For this review, take the finished solid that the model builds, in its own axes (mm). A direction names the side the tool comes from. Give positions to 0.01 mm unless a question says otherwise; leave off trailing zeros. Loops run counter-clockwise (first coordinate to the right, second up) from the corner with the lowest first, then second, coordinate; pieces in that order, holes last.
```python
from build123d import *

# Parameters (mm, degrees)
BASE_FLANGE1_START = -58.5
BASE_FLANGE1_DEPTH = 58.5
SKETCH7_R          = 3.2
CUT_EXTRUDE1_DEPTH = 75.505788366
SKETCH8_R          = 4.45
CUT_EXTRUDE2_DEPTH = 75.505788366


# Read off the part's stored shape, not the designer's step: Base-Flange1
with BuildPart() as part:
    # Base-Flange1 outline → Base-Flange1 (new body)
    with BuildSketch(Plane.XY.offset(BASE_FLANGE1_START)):
        with BuildLine():
            ThreePointArc((9.9634, 0), (11.7924024, 0.7575976), (12.55, 2.5866))
            Line((12.55, 2.5866), (12.55, 44.4))
            Line((12.55, 44.4), (10.7, 44.4))
            Line((10.7, 44.4), (10.7, 2.5866))
            ThreePointArc((10.7, 2.5866), (10.484254855, 2.065745145), (9.9634, 1.85))
            Line((9.9634, 1.85), (0, 1.85))
            Line((0, 1.85), (0, 0))
            Line((0, 0), (9.9634, 0))
        make_face()
    extrude(amount=BASE_FLANGE1_DEPTH)

    # Sketch7 → Cut-Extrude1 (cut, through all)
    with BuildSketch(Plane(origin=(0, 0, 0), x_dir=(0, 0, -1), z_dir=(1, 0, 0))):
        with BuildLine():
            Line((11.941667032, 43.361555933), (58.5, 17))
            Line((58.5, 17), (58.5, 44.4))
            Line((58.5, 44.4), (8, 44.4))
            ThreePointArc((8, 44.4), (10.038081516, 44.136034109), (11.941667032, 43.361555933))
        make_face()
        with BuildLine():
            ThreePointArc((0, 36.4), (2.343145751, 42.056854249), (8, 44.4))
            Line((8, 44.4), (0, 44.4))
            Line((0, 44.4), (0, 36.4))
        make_face()
        with Locations((9.2, 36.15)):
            Circle(SKETCH7_R)
    extrude(amount=CUT_EXTRUDE1_DEPTH, mode=Mode.SUBTRACT)

    # Sketch8 → Cut-Extrude2 (cut, through all)
    with BuildSketch(Plane(origin=(0, 0, 0), x_dir=(1, 0, 0), z_dir=(0, 1, 0))):
        with Locations((0, 12.5)):
            Circle(SKETCH8_R)
        with BuildLine():
            Line((-5.05, 49.4), (-5.05, 58.5))
            ThreePointArc((-5.05, 58.5), (0, 63.55), (5.05, 58.5))
            Line((5.05, 58.5), (5.05, 49.4))
            ThreePointArc((5.05, 49.4), (0, 44.35), (-5.05, 49.4))
        make_face()
    extrude(amount=CUT_EXTRUDE2_DEPTH, mode=Mode.SUBTRACT)

    # Mirror1: part across plane


with BuildPart() as part_1:
    add(part.part)
    add(part.part.mirror(Plane(origin=(0, 0, -58.5), x_dir=(0, 0, 1), z_dir=(1, 0, 0))))


solid = part_1.part
```
Item 1: Take a section at A-A on y = 9.5. Give the boundary of the cut face in (x, z).
Answer:
outline: (-12.55, -58.5) - (-10.7, -58.5) - (-10.7, 0) - (-12.55, 0) - close; (10.7, -58.5) - (12.55, -58.5) - (12.55, 0) - (10.7, 0) - close
Item 2: Take a section at C-C on z = -9.2. Give the boundary of the cut face in (x, y), and give its area (3 significant figures).
Answer:
outline: (-12.55, 2.59) arc R2.59 ccw to (-9.96, 0) - (-2.99, 0) - (-2.99, 1.85) - (-9.96, 1.85) arc R0.74 cw to (-10.7, 2.59) - (-10.7, 32.95) - (-12.55, 32.95) - close; (-12.55, 39.35) - (-10.7, 39.35) - (-10.7, 44.31) - (-12.55, 44.31) - close; (2.99, 0) - (9.96, 0) arc R2.59 ccw to (12.55, 2.59) - (12.55, 32.95) - (10.7, 32.95) - (10.7, 2.59) arc R0.74 cw to (9.96, 1.85) - (2.99, 1.85) - close; (10.7, 39.35) - (12.55, 39.35) - (12.55, 44.31) - (10.7, 44.31) - close
area: 166 mm2
Item 3: For L1, parallel to X at y = 5, z = -10; L2, parallel to Z at x = 0, y = 1.1; L3, parallel to Y at x = 11.7, z = -9.2, list the stretches that pass through material, from the lowest coordinate up.
Answer:
L1: x = -12.55 to -10.7, 10.7 to 12.55
L2: z = -44.35 to -16.95, -8.05 to 0
L3: y = 0.67 to 32.95, 39.35 to 44.31
Item 4: Tool access review of faces 5 (the flat face through (0, 1.85, -30)), 6 (the flat face through (-5.05, 1, -54)), 7 (the flat face through (11.61, 30.37, -34.89)): name each direction out of +Z, -Z, +X, -X, +Y, -Y from which nothing blocks a thin tool from reaching the whole face with its end or side.
Answer:
face 5: +Z, -Z, +Y
face 6: -Z, +Y, -Y
face 7: -Z, +X, -X, +Y
Item 5: Clearance check with flat-ended pins moving along their axes: pin 1 Ø8 at (x, z) = (0, -12.5) entering from +Y; pin 2 Ø0.9 at (y, z) = (1, -54) entering from -X; pin 3 Ø4 at (x, z) = (6.5, -16.5) entering from +Y; pin 4 Ø2 at (y, z) = (0.5, -53) entering from +X. State where each tip first meets the part, or that it passes through.
Answer:
pin 1: passes through
pin 2: stops at x = -12.29
pin 3: stops at y = 1.85
pin 4: stops at x = 12.31
Item 6: The part is to be moulded in two halves that separate along Z. For faces 1 (the cylindrical face through (11.612, 33.026, -8.506)), 2 (the flat face through (11, 16, 0)), 3 (the flat face through (-11, 7, -58.5)), 4 (the flat face through (5.05, 1, -54)), say which applies: released by +Z, released by -Z, zero draft, split by the parting line, or undercut.
Answer:
face 1: undercut
face 2: released by +Z
face 3: released by -Z
face 4: zero draft
Item 7: Take a section at B-B on x = 0. Give the boundary of the cut face in (y, z).
Answer:
outline: (0, -44.35) - (1.85, -44.35) - (1.85, -16.95) - (0, -16.95) - close; (0, -8.05) - (1.85, -8.05) - (1.85, 0) - (0, 0) - close
Item 8: Take a section at D-D on z = -32. Give the boundary of the cut face in (x, y), and give its area (3 significant figures).
Answer:
outline: (-12.55, 2.59) arc R2.59 ccw to (-9.96, 0) - (9.96, 0) arc R2.59 ccw to (12.55, 2.59) - (12.55, 32) - (10.7, 32) - (10.7, 2.59) arc R0.74 cw to (9.96, 1.85) - (-9.96, 1.85) arc R0.74 cw to (-10.7, 2.59) - (-10.7, 32) - (-12.55, 32) - close
area: 155 mm2
